```python
from build123d import *

# Parameters (mm, degrees)
SKETCH1_W           = 180
SKETCH1_H           = 100
BOSS_EXTRUDE1_DEPTH = 3
SKETCH2_R           = 1.6
CUT_EXTRUDE1_DEPTH  = 10
FILLET1_R           = 5
SKETCH3_R           = 1
SKETCH3_R_2         = 3.43
SKETCH3_R_3         = 1.4
SKETCH3_W           = 12
SKETCH3_H           = 22.5
CUT_EXTRUDE2_DEPTH  = 3


with BuildPart() as part:
    # Sketch1 → Boss-Extrude1 (new body)
    with BuildSketch(Plane(origin=(0, 0, 0), x_dir=(1, 0, 0), z_dir=(0, 1, 0))):
        Rectangle(SKETCH1_W, SKETCH1_H)
    extrude(amount=BOSS_EXTRUDE1_DEPTH)

    # Sketch2 → Cut-Extrude1 (cut)
    with BuildSketch(Plane(origin=(0, 3, 0), x_dir=(1, 0, 0), z_dir=(0, 1, 0))):
        with Locations(Location((-65, -20, 0), (0, 0, 270))):
            Circle(SKETCH2_R)
        with Locations(Location((-63.4, 28.3, 0), (0, 0, 270))):
            Circle(SKETCH2_R)
        with Locations(Location((-12.6, 13, 0), (0, 0, 270))):
            Circle(SKETCH2_R)
        with Locations(Location((-12.6, -14.9, 0), (0, 0, 270))):
            Circle(SKETCH2_R)
    extrude(amount=-CUT_EXTRUDE1_DEPTH, mode=Mode.SUBTRACT)

    # Fillet1
    fillet1_edges = [part.edges().sort_by_distance(p)[0] for p in [
        (90, 1.5, 50),
        (-90, 1.5, 50),
        (-90, 1.5, -50),
        (90, 1.5, -50),
    ]]
    fillet(fillet1_edges, radius=FILLET1_R)

    # Sketch3 → Cut-Extrude2 (cut)
    with BuildSketch(Plane(origin=(0, 3, 0), x_dir=(1, 0, 0), z_dir=(0, 1, 0))):
        with Locations(Location((69, 10.12, 0), (0, 0, 270))):
            Circle(SKETCH3_R)
        with Locations(Location((69, 37.38, 0), (0, 0, 270))):
            Circle(SKETCH3_R)
        with Locations(Location((69, -25, 0), (0, 0, 270))):
            Circle(SKETCH3_R_2)
        with Locations(Location((69, -5, 0), (0, 0, 270))):
            Circle(SKETCH3_R_2)
        with Locations(Location((42.5, 12.5, 0), (0, 0, 270))):
            Circle(SKETCH3_R_3)
        with Locations(Location((15, 12.5, 0), (0, 0, 270))):
            Circle(SKETCH3_R_3)
        with Locations(Location((28.75, 42, 0), (0, 0, 270))):
            Circle(SKETCH3_R_3)
        with Locations((69, 23.75)):
            Rectangle(SKETCH3_W, SKETCH3_H)
    extrude(amount=-CUT_EXTRUDE2_DEPTH, mode=Mode.SUBTRACT)


solid = part.part
```
Verification items for the finished model (mm, model axes). Coordinates: 2 decimals unless noted, no trailing zeros. Loops run counter-clockwise (first coordinate to the right, second up) from the corner with the lowest first, then second, coordinate; pieces in that order, holes last. Notation, with made-up numbers: (33, -13) -> (49, -13) arc R33 ccw to (49, 19) -> close; hole circle Ø11 at (34.25, -22.75). An arc over 180 degrees is marked (long way). Put each result on its own line as item: value.
1. Section check B-B, the plane y = 1.7. Give the number of separate pieces and of enclosed holes in the cut face, then the cut area to 3 significant figures.
Result set:
separate pieces: 1
enclosed holes: 12
area: 17,600 mm^2
2. Mould release check, pull along X, two halves, no side actions. Record for faces 1 (the face through (-89, 2, -48)), 2 (the face through (-1, 0, -1)), 3 (the face through (-64.96, 1.52, -28.65)): pulls with the +X half, pulls with the -X half, needs draft (parallel to the pull), parting line crosses it, or undercut.
Result set:
face 1: pulls with the -X half
face 2: needs draft
face 3: undercut
3. Section check A-A, the plane z = 5. Record the boundary of the cut face in (x, y), then the cut area to 3 significant figures.
Result set:
outline: (-90, 0) -> (65.57, 0) -> (65.57, 3) -> (-90, 3) -> close; (72.43, 0) -> (90, 0) -> (90, 3) -> (72.43, 3) -> close
area: 519 mm^2
4. Thickness scan on line 1 (X direction, y = 0.65, z = 5); line 2 (X direction, y = 2.9, z = -10); line 3 (X direction, y = 1.5, z = -13). Record the ranges inside material, lowest first.
Result set:
line 1: x = -90 to 65.57, 72.43 to 90
line 2: x = -90 to 68.01, 69.99 to 90
line 3: x = -90 to -14.2, -11 to 13.69, 16.31 to 41.19, 43.81 to 63, 75 to 90
